```python
from build123d import *

# Parameters (mm, degrees)
F0_R     = 4.375
F1_DEPTH = 50
F2_R     = 1.25
F3_DEPTH = 12.5
F4_R     = 2.25
F5_DEPTH = 5.001


with BuildPart() as f1:
    # F0 (on Top) → F1 (new body)
    with BuildSketch(Plane.XY):
        with BuildLine():
            Line((-2.375, -9.375), (0, -9.375))
            ThreePointArc((0, -9.375), (6.629126, 6.629126), (-9.375, 0))
            Line((-9.375, 0), (-9.375, -21.375))
            Line((-9.375, -21.375), (-4.375, -21.375))
            Line((-4.375, -21.375), (-4.375, -11.375))
            ThreePointArc((-4.375, -11.375), (-3.789214, -9.960786), (-2.375, -9.375))
        make_face()
        Circle(F0_R, mode=Mode.SUBTRACT)
    extrude(amount=F1_DEPTH)

    # F2 (on Right) → F3 (cut, symmetric)
    with BuildSketch(Plane.YZ):
        with Locations((0, 12.5)):
            Circle(F2_R)
        with Locations((0, 37.5)):
            Circle(F2_R)
    extrude(amount=F3_DEPTH, both=True, mode=Mode.SUBTRACT)

    # F4 (on face) → F5 (cut, through all)
    with BuildSketch(Plane.YZ.offset(-4.375)):
        with Locations((-16.375, 40)):
            Circle(F4_R)
        with Locations((-16.375, 10)):
            Circle(F4_R)
    extrude(amount=-F5_DEPTH, mode=Mode.SUBTRACT)


solid = f1.part
```
Work out the finished part from the listing and answer in its coordinate system (mm). A direction names the side the tool comes from. Coordinates: 2 decimals unless noted, no trailing zeros. Write each loop counter-clockwise with the first axis right and the second up, starting at its lowest first coordinate (ties: lowest second). Pieces come first, ordered by that corner, then holes.
Q1. Which of the six approach directions +Z, -Z, +X, -X, +Y, -Y give full straight-line access (tool end or side, diameter ignored) to faces 1 (the face through (-6.75, -0.16, 13.74)), 2 (the face through (-4.375, -16, 25))?
Q2. Find the intervals of material crossed by line 1 (Z direction, x = 5.95, y = 0); line 2 (X direction, y = -13.5, z = 33.5) (3 decimals); line 3 (X direction, y = 4, z = 15.5), in increasing order.
Q3. Each of these flat-tipped pins is pushed along its axis until it touches: pin 1 Ø7 at (x, y) = (0, 0) entering from +Z; pin 2 Ø5 at (x, z) = (1, 31.5) entering from -Y (3 decimals); pin 3 Ø1 at (y, z) = (-5.5, 6) entering from +X; pin 4 Ø5 at (y, z) = (-16.375, 40) entering from +X (3 decimals). Where does it stop, or does it pass through?
Q4. A cutting plane is placed at D-D, the plane x = 5. Give the vertices of the cut face in (y, z).
Q5. Determine the mould class of faces 3 (the face through (6.84, 6.41, 24.65)), 4 (the face through (-7, -21.375, 25)), 5 (the face through (6.82, -0.27, 36.28)) for opening direction Y: released by +Y, released by -Y, zero draft, split by the parting line, or undercut.
Q6. A cutting plane is placed at A-A, the plane z = 10. Give the vertices of the cut face in (x, y) (3 decimals), then the cut area to 3 significant figures.
Q7. A cutting plane is placed at C-C, the plane z = 39.5. Give the vertices of the cut face in (x, y) (3 decimals), then the cut area to 3 significant figures.
Q8. A cutting plane is placed at B-B, the plane x = -3.5. Give the vertices of the cut face in (y, z) (3 decimals), then the cut area to 3 significant figures.
Findings below:
1. face 1: +X, -X
1. face 2: +Z, -Z, +X, -Y
2. line 1: z = 0 to 11.25, 13.75 to 36.25, 38.75 to 50
2. line 2: x = -9.375 to -4.375
2. line 3: x = -8.48 to -1.77, 1.77 to 8.48
3. pin 1: passes through
3. pin 2: stops at y = -9.375
3. pin 3: stops at x = 7.93
3. pin 4: stops at x = -4.375
4. outline: (-7.93, 0) - (7.93, 0) - (7.93, 50) - (-7.93, 50) - close; hole circle Ø2.5 at (0, 12.5); hole circle Ø2.5 at (0, 37.5)
5. face 3: split by the parting line
5. face 4: released by -Y
5. face 5: undercut
6. outline: (-9.375, -21.375) - (-4.375, -21.375) - (-4.375, -18.625) - (-9.375, -18.625) - close; (-9.375, -14.125) - (-4.375, -14.125) - (-4.375, -11.375) arc R2 cw to (-2.375, -9.375) - (0, -9.375) arc R9.375 ccw (long way) to (-9.375, 0) - close; hole circle Ø8.75 at (0, 0)
6. area: 273 mm2
7. outline: (-9.375, -21.375) - (-4.375, -21.375) - (-4.375, -18.569) - (-9.375, -18.569) - close; (-9.375, -14.181) - (-4.375, -14.181) - (-4.375, -11.375) arc R2 cw to (-2.375, -9.375) - (0, -9.375) arc R9.375 ccw (long way) to (-9.375, 0) - close; hole circle Ø8.75 at (0, 0)
7. area: 274 mm2
8. outline: (-9.721, 0) - (-2.625, 0) - (-2.625, 50) - (-9.721, 50) - close; (2.625, 0) - (8.697, 0) - (8.697, 50) - (2.625, 50) - close
8. area: 658 mm2
